Design review of the part built by this model. Coordinates are the model's own, in mm. A direction names the side the tool comes from. Round coordinates to 2 decimals unless told otherwise and drop trailing zeros. Write each loop counter-clockwise with the first axis right and the second up, starting at its lowest first coordinate (ties: lowest second). Pieces come first, ordered by that corner, then holes. Notation, with made-up numbers: (35.5, 75.5) - (62.5, 75.5) arc R23 ccw to (62.5, 83.5) - close; hole circle Ø6 at (46.25, 41). An arc over 180 degrees is marked (long way). Use one line per item in the form item = value.
```python
from build123d import *

# Parameters (mm, degrees)
PAD_DEPTH    = 31.8
SKETCH001_R  = 0.9
PAD001_DEPTH = 11.8


with BuildPart() as part:
    # Sketch → Pad (new body)
    with BuildSketch(Plane.XZ):
        with BuildLine():
            Line((0, 15), (14, 15))
            ThreePointArc((14, 0), (17, 7.5), (14, 15))
            Line((14, 0), (0, 0))
            ThreePointArc((0, 15), (-3, 7.5), (0, 0))
        make_face()
    extrude(amount=PAD_DEPTH)

    # Sketch001 (on Face6 of Pad) → Pad001 (join)
    with BuildSketch(Plane.XZ.offset(31.8)):
        with Locations((7, 7.5)):
            Circle(SKETCH001_R)
    extrude(amount=PAD001_DEPTH)


solid = part.part
```
Q1. We need section B-B on z = 7.5. Write out the cut boundary in (x, y).
Calculated:
outline = (-3, -31.8) - (6.1, -31.8) - (6.1, -43.6) - (7.9, -43.6) - (7.9, -31.8) - (17, -31.8) - (17, 0) - (-3, 0) - close
Q2. For P1, Ø1.5, axis at x = 10, z = 10, coming from the +Y side; P2, Ø2, axis at y = -5.5, z = 11.5, coming from the +X side; P3, Ø8, axis at y = -5, z = 13, coming from the -X side; P4, Ø10, axis at x = 4, y = -37.5, coming from the -Z side, all flat-tipped, find the tip position at first contact; note any pin that passes through.
Calculated:
P1 = 0
P2 = 16.58
P3 = -2.9
P4 = 6.6
Q3. We need section A-A on x = 7. Write out the cut boundary in (y, z), then the cut area to 3 significant figures.
Calculated:
outline = (-43.6, 6.6) - (-31.8, 6.6) - (-31.8, 0) - (0, 0) - (0, 15) - (-31.8, 15) - (-31.8, 8.4) - (-43.6, 8.4) - close
area = 498 mm2
Q4. To check wall thickness, follow line 1 along Y through (x, z) = (2.75, 6.75); line 2 along X through (y, z) = (-14, 11.5); line 3 along Z through (x, y) = (-1.75, -23). State the ranges of each line that lie inside material, in increasing order. Write a range as from..to.
Calculated:
line_1 = -31.8..0
line_2 = -2.24..16.24
line_3 = 2.44..12.56
Q5. Machinability: for faces 1 (the cylindrical face through (17, -15.7, 7.4)), 2 (the cylindrical face through (7.48, -37.62, 8.26)), which of the approach directions +Z, -Z, +X, -X, +Y, -Y give a long, thin tool a straight path to every point of the face, cutting with its end or side? Answer none if there is none.
Calculated:
face_1 = +X, +Y, -Y
face_2 = -Y
Q6. We need section C-C on y = -18. Write out the cut boundary in (x, z) (3 decimals), then the cut area to 3 significant figures.
Calculated:
outline = (0, 0) - (14, 0) arc R10.875 ccw to (14, 15) - (0, 15) arc R10.875 ccw to start
area = 272 mm2
Q7. We need section D-D on x = 13.25. Write out the cut boundary in (y, z).
Calculated:
outline = (-31.8, 0) - (0, 0) - (0, 15) - (-31.8, 15) - close
